```python
from build123d import *

# Parameters (mm, degrees)
F0_W     = 80.216743052
F0_H     = 56.6479042172
F1_DEPTH = 25.4
F2_DEPTH = 22.86
F3_DEPTH = 27.94
F4_DEPTH = 27.94


# Not quite as in the source:
# - the program builds the solid bodies; features that only make, move or delete a surface that nothing else refers to are left out


with BuildPart() as f1:
    # F0 (on Front) → F1 (new body)
    with BuildSketch(Plane.XZ):
        Polygon((-48.5848858953, 32.4588380754), (-48.5848858953, -32.4588380754), (48.5848858953, -32.4588380754), (48.5848858953, 32.4588380754), (23.2139006257, 32.4588380754), align=None)
        Polygon((45.9382493502, -7.469226185), (44.9628157303, -7.7861637805), (43.9371841267, -7.7861637805), (42.9617505067, -7.469226185), (42.1319971095, -6.8663750542), (41.5291459786, -6.0366216569), (41.2122083831, -5.061188037), (41.2122083831, -4.0355564333), (41.5291459786, -3.0601228134), (42.1319971095, -2.2303694161), (42.9617505067, -1.6275182853), (43.9371841267, -1.3105806898), (44.9628157303, -1.3105806898), (45.9382493502, -1.6275182853), (46.7680027475, -2.2303694161), (47.3708538784, -3.0601228134), (47.6877914738, -4.0355564333), (47.6877914738, -5.061188037), (47.3708538784, -6.0366216569), (46.7680027475, -6.8663750542), align=None, mode=Mode.SUBTRACT)
        Rectangle(F0_W, F0_H, mode=Mode.SUBTRACT)
        Polygon((46.129602097, 4.9471233192), (45.03331964, 4.5481091365), (43.8666802169, 4.5481091365), (42.77039776, 4.9471233192), (41.8767001128, 5.6970246853), (41.2933804012, 6.7073640628), (41.0907955914, 7.8562796116), (41.2933804012, 9.0051951604), (41.8767001128, 10.0155345378), (42.77039776, 10.765435904), (43.8666802169, 11.1644500867), (45.03331964, 11.1644500867), (46.129602097, 10.765435904), (47.0232997442, 10.0155345378), (47.6066194557, 9.0051951604), (47.8092042655, 7.8562796116), (47.6066194557, 6.7073640628), (47.0232997442, 5.6970246853), align=None, mode=Mode.SUBTRACT)
    extrude(amount=F1_DEPTH)

    # F0 (on Front) → F2 (join)
    with BuildSketch(Plane.XZ):
        Rectangle(F0_W, F0_H)
    extrude(amount=F2_DEPTH)

    # F0 (on Front) → F3 (join)
    with BuildSketch(Plane.XZ):
        Polygon((43.8666802169, 4.5481091365), (45.03331964, 4.5481091365), (46.129602097, 4.9471233192), (47.0232997442, 5.6970246853), (47.6066194557, 6.7073640628), (47.8092042655, 7.8562796116), (47.6066194557, 9.0051951604), (47.0232997442, 10.0155345378), (46.129602097, 10.765435904), (45.03331964, 11.1644500867), (43.8666802169, 11.1644500867), (42.77039776, 10.765435904), (41.8767001128, 10.0155345378), (41.2933804012, 9.0051951604), (41.0907955914, 7.8562796116), (41.2933804012, 6.7073640628), (41.8767001128, 5.6970246853), (42.77039776, 4.9471233192), align=None)
    extrude(amount=F3_DEPTH)

    # F0 (on Front) → F4 (join)
    with BuildSketch(Plane.XZ):
        Polygon((43.9371841267, -7.7861637805), (44.9628157303, -7.7861637805), (45.9382493502, -7.469226185), (46.7680027475, -6.8663750542), (47.3708538784, -6.0366216569), (47.6877914738, -5.061188037), (47.6877914738, -4.0355564333), (47.3708538784, -3.0601228134), (46.7680027475, -2.2303694161), (45.9382493502, -1.6275182853), (44.9628157303, -1.3105806898), (43.9371841267, -1.3105806898), (42.9617505067, -1.6275182853), (42.1319971095, -2.2303694161), (41.5291459786, -3.0601228134), (41.2122083831, -4.0355564333), (41.2122083831, -5.061188037), (41.5291459786, -6.0366216569), (42.1319971095, -6.8663750542), (42.9617505067, -7.469226185), align=None)
    extrude(amount=F4_DEPTH)


solid = f1.part
```
Design review of the part built by this model. Coordinates are the model's own, in mm. A direction names the side the tool comes from. Give positions to 0.01 mm unless a question says otherwise; leave off trailing zeros. Order: outer loops, then holes, each group sorted by start corner. A loop starts at its lowest first (then second) coordinate and runs counter-clockwise, first axis right, second up. Notation, with made-up numbers: (3, 60) -> (8, 60) arc R4 cw to (8, 64) -> close; hole circle Ø11 at (31, 20.5). An arc over 180 degrees is marked (long way). Write each question's results on one line, items separated by ' | '. Start each with the question number.
Q1. Add section B-B on z = -26.5. Give the boundary of the cut face in (x, y).
Q2. Mouldability with a two-part tool opening along Z and no side actions: class faces 3 (the flat face through (-1, -22.86, 0)), 4 (the flat face through (44, -27.94, -5)), 5 (the flat face through (-1, -13, -32.459)), 6 (the flat face through (1, -13, 32.459)) as +Z half, -Z half, draft (parallel to the pull), parting line (faces both ways), or undercut.
Q3. Machinability: for faces 1 (the flat face through (-1, -24, -28.324)), 2 (the flat face through (-48.585, -13, 0)), which of the approach directions +Z, -Z, +X, -X, +Y, -Y give a long, thin tool a straight path to every point of the face, cutting with its end or side? Answer none if there is none.
Q4. For pin 1 (1.1 mm diameter, centred on y = -26, z = -4.5, fed in from -X); pin 2 (0.8 mm diameter, centred on y = -27.5, z = -4.5, fed in from +X); pin 3 (1.1 mm diameter, centred on x = 44, y = -27, fed in from -Z), all flat-tipped, find the tip position at first contact; note any pin that passes through.
Q5. Wall thickness on L1, parallel to X at y = -23, z = -4; L2, parallel to Y at x = -9.5, z = 0; L3, parallel to Z at x = 10, y = -25.25: over which ranges is each line inside the solid? List them lowest first. Write a range as from..to.
Q6. Add section A-A on x = -7.5. Give the boundary of the cut face in (y, z).
Found:
1) outline: (-48.58, -25.4) -> (-40.11, -25.4) -> (-40.11, -22.86) -> (40.11, -22.86) -> (40.11, -25.4) -> (48.58, -25.4) -> (48.58, 0) -> (-48.58, 0) -> close
2) face 3: undercut | face 4: draft | face 5: -Z half | face 6: +Z half
3) face 1: -Y | face 2: +Z, -Z, -X, +Y, -Y
4) pin 1: stops at x = 41.21 | pin 2: stops at x = 47.69 | pin 3: stops at z = -7.79
5) L1: x = -48.58..-40.11, 40.11..48.58 | L2: y = -22.86..0 | L3: z = -32.46..-28.32, 28.32..32.46
6) outline: (-25.4, -32.46) -> (0, -32.46) -> (0, 32.46) -> (-25.4, 32.46) -> (-25.4, 28.32) -> (-22.86, 28.32) -> (-22.86, -28.32) -> (-25.4, -28.32) -> close
